from build123d import *

# Parameters (mm, degrees)
EXTRUDE1_DEPTH     = 3.175
SKETCH2_R          = 3.302
CUT_EXTRUDE1_DEPTH = 3.175


with BuildPart() as part:
    # Sketch1 → Extrude1 (new body)
    with BuildSketch(Plane.XY):
        Polygon((3.175, 9.525), (6.35, 9.525), (6.35, 3.175), (9.525, 3.175), (9.525, -3.175), (6.35, -3.175), (6.35, -9.525), (3.175, -9.525), (3.175, -12.7), (-3.175, -12.7), (-3.175, -9.525), (-6.35, -9.525), (-6.35, -3.175), (-9.525, -3.175), (-9.525, 3.175), (-6.35, 3.175), (-6.35, 9.525), (-3.175, 9.525), (-3.175, 12.7), (3.175, 12.7), align=None)
    extrude(amount=EXTRUDE1_DEPTH)

    # Sketch2 → Cut-Extrude1 (cut)
    with BuildSketch(Plane(origin=(0, 0, 0), x_dir=(-1, 0, 0), z_dir=(0, 0, -1))):
        Circle(SKETCH2_R)
    extrude(amount=-CUT_EXTRUDE1_DEPTH, mode=Mode.SUBTRACT)


solid = part.part
The model under review builds one solid part; all positions refer to its coordinate system, in mm. A direction names the side the tool comes from. Give positions to 0.01 mm unless a question says otherwise; leave off trailing zeros. Order: outer loops, then holes, each group sorted by start corner. A loop starts at its lowest first (then second) coordinate and runs counter-clockwise, first axis right, second up. Notation, with made-up numbers: (6.5, 8.25) -> (10.5, 8.25) arc R22 cw to (10.5, 20.25) -> close; hole circle Ø9 at (83, 49). An arc over 180 degrees is marked (long way). Write item = value, one per line. Start each with the question number.
(1) For L1, parallel to Y at x = 0, z = 0.7; L2, parallel to X at y = -8.25, z = 2.2; L3, parallel to Y at x = -6.5, z = 2.9 (3 decimals), list the stretches that pass through material, from the lowest coordinate up. Write a range as from..to.
(2) For pin 1 Ø1.6 at (x, z) = (-7.5, 1) entering from +Y (3 decimals); pin 2 Ø1 at (y, z) = (6, 1.5) entering from -X; pin 3 Ø1 at (y, z) = (10.5, 2.5) entering from -X (3 decimals), all flat-tipped, find the tip position at first contact; note any pin that passes through.
(3) Take a section at A-A (y = 0). Write out the cut boundary in (x, z) (3 decimals), plus the area to 3 significant figures.
(4) Take a section at B-B (x = 0). Write out the cut boundary in (y, z) (3 decimals).
(5) Take a section at D-D (y = -10.75). Write out the cut boundary in (x, z) (3 decimals).
(6) Take a section at C-C (z = 2.3). Write out the cut boundary in (x, y) (3 decimals), plus the area to 3 significant figures.
(7) Tool access review of faces 4 (the flat face through (5, 9.525, 2)), 5 (the flat face through (0, -12.7, 2)), 6 (the flat face through (-3.175, -11, 2)), 7 (the flat face through (-3.175, 11, 2)), 8 (the flat face through (8, -3.175, 2)): name each direction out of +Z, -Z, +X, -X, +Y, -Y from which nothing blocks a thin tool from reaching the whole face with its end or side.
(8) Draft analysis for pull direction X (two halves, no side actions). For faces 1 (the flat face through (6.35, -6, 2)), 2 (the flat face through (8, 3.175, 2)), 3 (the flat face through (-9.525, 0, 2)), state which applies: +X half, -X half, draft (parallel to the pull), parting line (faces both ways), or undercut.
Returned:
q1.L1 = -12.7..-3.3, 3.3..12.7
q1.L2 = -6.35..6.35
q1.L3 = -3.175..3.175
q2.pin_1 = 3.175
q2.pin_2 = -6.35
q2.pin_3 = -3.175
q3.outline = (-9.525, 0) -> (-3.302, 0) -> (-3.302, 3.175) -> (-9.525, 3.175) -> close; (3.302, 0) -> (9.525, 0) -> (9.525, 3.175) -> (3.302, 3.175) -> close
q3.area = 39.5 mm²
q4.outline = (-12.7, 0) -> (-3.302, 0) -> (-3.302, 3.175) -> (-12.7, 3.175) -> close; (3.302, 0) -> (12.7, 0) -> (12.7, 3.175) -> (3.302, 3.175) -> close
q5.outline = (-3.175, 0) -> (3.175, 0) -> (3.175, 3.175) -> (-3.175, 3.175) -> close
q6.outline = (-9.525, -3.175) -> (-6.35, -3.175) -> (-6.35, -9.525) -> (-3.175, -9.525) -> (-3.175, -12.7) -> (3.175, -12.7) -> (3.175, -9.525) -> (6.35, -9.525) -> (6.35, -3.175) -> (9.525, -3.175) -> (9.525, 3.175) -> (6.35, 3.175) -> (6.35, 9.525) -> (3.175, 9.525) -> (3.175, 12.7) -> (-3.175, 12.7) -> (-3.175, 9.525) -> (-6.35, 9.525) -> (-6.35, 3.175) -> (-9.525, 3.175) -> close; hole circle Ø6.604 at (0, 0)
q6.area = 288 mm²
q7.face_4 = +Z, -Z, +X, +Y
q7.face_5 = +Z, -Z, +X, -X, -Y
q7.face_6 = +Z, -Z, -X, -Y
q7.face_7 = +Z, -Z, -X, +Y
q7.face_8 = +Z, -Z, +X, -Y
q8.face_1 = +X half
q8.face_2 = draft
q8.face_3 = -X half
